Verification items for the finished model (mm, model axes). A direction names the side the tool comes from. Give positions to 0.01 mm unless a question says otherwise; leave off trailing zeros. Loops run counter-clockwise (first coordinate to the right, second up) from the corner with the lowest first, then second, coordinate; pieces in that order, holes last. Notation, with made-up numbers: M 78.25,44 L 121.25,44 A17 ccw 121.25,73 Z; hole C 36,41 d4. An arc over 180 degrees is marked long. Use a Markdown table: item, result.
from build123d import *

# Parameters (mm, degrees)
F0_W     = 6
F0_H     = 6
F0_R     = 1.6
F1_DEPTH = 4
F2_DEPTH = 9


with BuildPart() as f1:
    # F0 (on Top) → F1 (new body)
    with BuildSketch(Plane.XY):
        Rectangle(F0_W, F0_H)
        Circle(F0_R, mode=Mode.SUBTRACT)
        Circle(F0_R)
    extrude(amount=-F1_DEPTH)

    # F0 (on Top) → F2 (join)
    with BuildSketch(Plane.XY):
        Circle(F0_R)
    extrude(amount=F2_DEPTH)


solid = f1.part
(1) Gauge pin test, flat end, axial feed: P1, Ø2, axis at x = 1, z = 4.5, coming from the -Y side. Record the tip position at first contact, or that the pin passes through.
Results below:
| item | result |
|---|---|
| P1 | y = -1.6 |
(2) Cross-section at A-A on y = 0. Record the cut outline in (x, z), then the cut area to 3 significant figures.
Results below:
| item | result |
|---|---|
| outline | M -3,-4 L 3,-4 L 3,0 L 1.6,0 L 1.6,9 L -1.6,9 L -1.6,0 L -3,0 Z |
| area | 52.8 mm^2 |
(3) Material ranges on line 1 (Z direction, x = 2.5, y = 0.05); line 2 (X direction, y = 0.6, z = 0.25); line 3 (Y direction, x = 1.3, z = 5.5), recorded low to high.
Results below:
| item | result |
|---|---|
| line 1 | -4 to 0 |
| line 2 | -1.48 to 1.48 |
| line 3 | -0.93 to 0.93 |
(4) Set-up check for faces 1 (the flat face through (1.3, 1.4, 0)), 2 (the flat face through (0, 0, -4)): record each of +Z, -Z, +X, -X, +Y, -Y from which the full face is reachable in a straight line by a thin tool's end or side.
Results below:
| item | result |
|---|---|
| face 1 | +Z |
| face 2 | -Z, +X, -X, +Y, -Y |
(5) Cross-section at C-C on z = 4.75. Record the cut outline in (x, y), then the cut area to 3 significant figures.
Results below:
| item | result |
|---|---|
| outline | C 0,0 d3.2 |
| area | 8.04 mm^2 |
(6) Cross-section at D-D on y = -2.2. Record the cut outline in (x, z), then the cut area to 3 significant figures.
Results below:
| item | result |
|---|---|
| outline | M -3,-4 L 3,-4 L 3,0 L -3,0 Z |
| area | 24.0 mm^2 |
